Design review of the part built by this model. Coordinates are the model's own, in mm. Round coordinates to 2 decimals unless told otherwise and drop trailing zeros. Return JSON: item names as keys, results as strings. Group by question number.
(1) Clearance check with flat-ended pins moving along their axes: pin 1 (1.2 mm diameter, centred on x = 368, z = 2, fed in from -Y); pin 2 (1.2 mm diameter, centred on y = 7, z = 2, fed in from -X); pin 3 (2.5 mm diameter, centred on x = 7.5, y = 46.18, fed in from +Z); pin 4 (2 mm diameter, centred on y = 8, z = 2, fed in from +X). State where each tip first meets the part, or that it passes through.
(2) Wall thickness on L1, parallel to X at y = 150.5, z = 2.4; L2, parallel to Y at x = 58.5, z = 0.8; L3, parallel to Y at x = 7.5, z = 1.7: over which ranges is each line inside the solid? List them lowest first. Write a range as [from, to].
(3) We need section A-A, the plane z = 3.15. Give the number of separate pieces and of enclosed holes in the cut face, and give its area (3 significant figures).
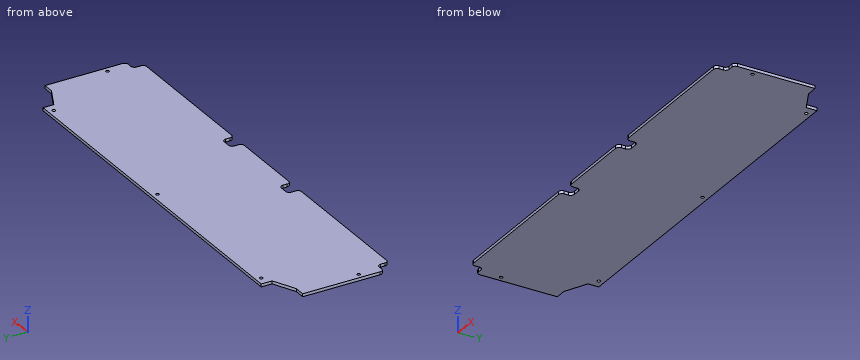
from build123d import *

# Parameters (mm, degrees)
SKETCH_1_W          = 600
SKETCH_1_H          = 158
EXTRUDE_1_DEPTH     = 4
SKETCH_2_W          = 20
SKETCH_2_H          = 16
SKETCH_2_W_2        = 16
CUT_EXTRUDE_1_DEPTH = 10
FILLET_1_R          = 5
HOLE_WIZARD_M4_1_D  = 4.5


with BuildPart() as part:
    # ｽｹｯﾁ1 → ﾎﾞｽ - 押し出し1 (new body)
    with BuildSketch(Plane.XY):
        with Locations((300, 79)):
            Rectangle(SKETCH_1_W, SKETCH_1_H)
    extrude(amount=EXTRUDE_1_DEPTH)

    # ｽｹｯﾁ2 → ｶｯﾄ - 押し出し1 (cut)
    with BuildSketch(Plane.XY.offset(4)):
        Polygon((46, 158), (46, 143), (15, 128), (0, 128), (0, 158), align=None)
        Polygon((600, 158), (600, 128), (585, 128), (554, 143), (554, 158), align=None)
        with Locations((366.5, 8)):
            Rectangle(SKETCH_2_W, SKETCH_2_H)
        with Locations((8, 8)):
            Rectangle(SKETCH_2_W_2, SKETCH_2_H)
        with Locations((233.5, 8)):
            Rectangle(SKETCH_2_W, SKETCH_2_H)
        with Locations((592, 8)):
            Rectangle(SKETCH_2_W_2, SKETCH_2_H)
    extrude(amount=-CUT_EXTRUDE_1_DEPTH, mode=Mode.SUBTRACT)

    # ﾌｨﾚｯﾄ1
    fillet_1_edges = [part.edges().sort_by_distance(p)[0] for p in [
        (376.5, 0, 2),
        (356.5, 0, 2),
        (356.5, 16, 2),
        (376.5, 16, 2),
        (223.5, 0, 2),
        (223.5, 16, 2),
        (243.5, 16, 2),
        (243.5, 0, 2),
        (0, 16, 2),
        (16, 16, 2),
        (16, 0, 2),
        (584, 16, 2),
        (600, 16, 2),
        (584, 0, 2),
    ]]
    fillet(fillet_1_edges, radius=FILLET_1_R)

    # M4 すきま穴1 (through all)
    with Locations(Plane.XY.offset(4)):
        with Locations((58.5, 150.5), (300, 150.5), (541.5, 150.5), (592.5, 46.18), (7.5, 46.18)):
            Hole(HOLE_WIZARD_M4_1_D / 2)


solid = part.part
Solutions:
{
 "1": {"pin 1": "y = 16", "pin 2": "x = 16", "pin 3": "through", "pin 4": "x = 584"},
 "2": {"L1": "[46, 56.25], [60.75, 297.75], [302.25, 539.25], [543.75, 554]", "L2": "[0, 148.25], [152.75, 158]", "L3": "[16, 43.93], [48.43, 128]"},
 "3": {"separate pieces": "1", "enclosed holes": "5", "area": "91,300 mm^2"}
}
